```python
from build123d import *

# Parameters (mm, degrees)
SKETCH1_W                                          = 41.91
SKETCH1_H                                          = 101.6
BOSS_EXTRUDE1_DEPTH                                = 41.275
CUT_EXTRUDE6_DEPTH                                 = 78.72202857
SKETCH3_R                                          = 14.3002
CUT_EXTRUDE2_DEPTH                                 = 69.726833551
SKETCH17_W                                         = 28.321
SKETCH17_H                                         = 10.16
CUT_EXTRUDE7_DEPTH                                 = 78.72202857
SKETCH4_R                                          = 3.2258
CUT_EXTRUDE3_DEPTH                                 = 112.648097386
FILLET2_R                                          = 3.175
CSK_FOR_10_FLAT_HEAD_MACHINE_SCREW_100_D           = 5.6134
CSK_FOR_10_FLAT_HEAD_MACHINE_SCREW_100_DEPTH       = 38.1
CSK_FOR_10_FLAT_HEAD_MACHINE_SCREW_100_CSINK_D     = 9.779
CSK_FOR_10_FLAT_HEAD_MACHINE_SCREW_100_CSINK_ANGLE = 100
CSK_FOR_10_FLAT_HEAD_MACHINE_SCREW_100_TIP         = 1.686435499
FILLET3_R                                          = 2.54
FILLET4_R                                          = 1.27


with BuildPart() as part:
    # Sketch1 → Boss-Extrude1 (new body)
    with BuildSketch(Plane(origin=(0, 0, 0), x_dir=(1, 0, 0), z_dir=(0, 1, 0))):
        Rectangle(SKETCH1_W, SKETCH1_H)
    extrude(amount=BOSS_EXTRUDE1_DEPTH)

    # Sketch13 → Cut-Extrude6 (cut, through all)
    with BuildSketch(Plane.ZY.offset(20.955)):
        Polygon((-6.872463407, 34.925), (-12.7, 26.60241523), (-12.7, 13.632261674), (-7.600905481, 6.35), (50.8, 6.35), (50.8, 34.925), align=None)
    extrude(amount=-CUT_EXTRUDE6_DEPTH, mode=Mode.SUBTRACT)

    # Sketch3 → Cut-Extrude2 (cut, through all)
    # profile 1 of 2: a face of its own
    with BuildSketch(Plane(origin=(0, 41.275, 0), x_dir=(1, 0, 0), z_dir=(0, 1, 0))):
        with Locations(Location((0, -25.4, 0), (0, 0, 270))):
            Circle(SKETCH3_R)
        Polygon((5.499261314, -25.4), (2.749630657, -20.6375), (-2.749630657, -20.6375), (-5.499261314, -25.4), (-2.749630657, -30.1625), (2.749630657, -30.1625), align=None, mode=Mode.SUBTRACT)
    # profile 2 of 2: a face of its own
    with BuildSketch(Plane(origin=(0, 41.275, 0), x_dir=(1, 0, 0), z_dir=(0, 1, 0))):
        Polygon((2.749630657, -30.1625), (5.499261314, -25.4), (2.749630657, -20.6375), (-2.749630657, -20.6375), (-5.499261314, -25.4), (-2.749630657, -30.1625), align=None)
    extrude(amount=-CUT_EXTRUDE2_DEPTH, mode=Mode.SUBTRACT)

    # Sketch17 → Cut-Extrude7 (cut, through all)
    with BuildSketch(Plane.ZY.offset(20.955)):
        with Locations((-36.6395, 5.08)):
            Rectangle(SKETCH17_W, SKETCH17_H)
    extrude(amount=-CUT_EXTRUDE7_DEPTH, mode=Mode.SUBTRACT)

    # Sketch4 → Cut-Extrude3 (cut, through all)
    with BuildSketch(Plane(origin=(0, 0, -50.8), x_dir=(-1, 0, 0), z_dir=(0, 0, -1))):
        with Locations((11.1125, 20.6375)):
            Circle(SKETCH4_R)
        with Locations((-11.1125, 20.6375)):
            Circle(SKETCH4_R)
    extrude(amount=-CUT_EXTRUDE3_DEPTH, mode=Mode.SUBTRACT)

    # Fillet2
    fillet2_edges = [part.edges().sort_by_distance(p)[0] for p in [
        (20.955, 3.175, 50.8),
        (-20.955, 3.175, 50.8),
        (0, 10.16, -50.8),
        (0, 10.16, -22.479),
        (0, 0, -22.479),
        (20.955, 38.1, 50.8),
        (-20.955, 38.1, 50.8),
    ]]
    fillet(fillet2_edges, radius=FILLET2_R)

    # CSK for #10 Flat Head Machine Screw (100)4
    with Locations(Plane.XY.offset(-12.7)):
        with Locations((-11.1125, 20.6375), (11.1125, 20.6375)):
            CounterSinkHole(CSK_FOR_10_FLAT_HEAD_MACHINE_SCREW_100_D / 2, CSK_FOR_10_FLAT_HEAD_MACHINE_SCREW_100_CSINK_D / 2, depth=CSK_FOR_10_FLAT_HEAD_MACHINE_SCREW_100_DEPTH, counter_sink_angle=CSK_FOR_10_FLAT_HEAD_MACHINE_SCREW_100_CSINK_ANGLE)
            with Locations((0, 0, -(CSK_FOR_10_FLAT_HEAD_MACHINE_SCREW_100_DEPTH + CSK_FOR_10_FLAT_HEAD_MACHINE_SCREW_100_TIP / 2))):  # 118° drill point
                Cone(0, CSK_FOR_10_FLAT_HEAD_MACHINE_SCREW_100_D / 2, CSK_FOR_10_FLAT_HEAD_MACHINE_SCREW_100_TIP, mode=Mode.SUBTRACT)

    # Fillet3
    fillet3_edges = [part.edges().sort_by_distance(p)[0] for p in [
        (0, 34.925, -6.872463407),
        (0, 6.35, -7.600905481),
    ]]
    fillet(fillet3_edges, radius=FILLET3_R)

    # Fillet4
    fillet4_edges = [part.edges().sort_by_distance(p)[0] for p in [
        (0, 13.632261674, -12.7),
        (0, 26.60241523, -12.7),
    ]]
    fillet(fillet4_edges, radius=FILLET4_R)


solid = part.part
```
Input: part model. Units: mm. Frame: model coordinates. A direction names the side the tool comes from. Give positions to 0.01 mm unless a question says otherwise; leave off trailing zeros. Loops run counter-clockwise (first coordinate to the right, second up) from the corner with the lowest first, then second, coordinate; pieces in that order, holes last.
1) Line query: L1, parallel to X at y = 3, z = 25 (3 decimals); L2, parallel to Y at x = 17, z = 23.5 (3 decimals); L3, parallel to Y at x = -11, z = -38 (3 decimals). Output: solid intervals per line, ascending.
A:
L1: x = -20.955 to -14.295, 14.295 to 20.955
L2: y = 0 to 6.35, 34.925 to 41.275
L3: y = 10.16 to 17.414, 23.861 to 41.275
2) Section query B-B on x = 0. Return the cut outline in (y, z) (3 decimals).
A:
outline: (0, -19.304) arc R3.175 ccw to (3.175, -22.479) - (6.985, -22.479) arc R3.175 cw to (10.16, -25.654) - (10.16, -47.625) arc R3.175 ccw to (13.335, -50.8) - (41.275, -50.8) - (41.275, 11.1) - (34.925, 11.1) - (34.925, -5.55) arc R2.54 cw to (33.842, -7.631) - (26.93, -12.47) arc R1.27 cw to (26.202, -12.7) - (14.033, -12.7) arc R1.27 cw to (13.304, -12.47) - (7.433, -8.359) arc R2.54 cw to (6.35, -6.279) - (6.35, 11.1) - (0, 11.1) - close; (0, 39.7) - (6.35, 39.7) - (6.35, 50.8) - (0, 50.8) - close; (34.925, 39.7) - (41.275, 39.7) - (41.275, 50.8) - (34.925, 50.8) - close
3) Section query A-A on z = 5.5. Return the cut outline in (x, y) (3 decimals), and give its area (3 significant figures).
A:
outline: (-20.955, 0) - (20.955, 0) - (20.955, 6.35) - (-20.955, 6.35) - close; (-20.955, 34.925) - (20.955, 34.925) - (20.955, 41.275) - (-20.955, 41.275) - close
area: 532 mm2
4) Reachability of faces 4 (the cylindrical face through (0.293, 9.205, -23.384)), 5 (the cylindrical face through (0.293, 6.645, -7.467)) from +Z, -Z, +X, -X, +Y, -Y: full face, straight path, thin tool, end or side. Return the list, or none.
A:
face 4: -Z, +X, -X, -Y
face 5: +Z, +X, -X
5) Section query D-D on z = 25.4. Return the cut outline in (x, y) (3 decimals).
A:
outline: (-20.955, 0) - (-14.3, 0) - (-14.3, 6.35) - (-20.955, 6.35) - close; (-20.955, 34.925) - (-14.3, 34.925) - (-14.3, 41.275) - (-20.955, 41.275) - close; (14.3, 0) - (20.955, 0) - (20.955, 6.35) - (14.3, 6.35) - close; (14.3, 34.925) - (20.955, 34.925) - (20.955, 41.275) - (14.3, 41.275) - close
6) Contact query for flat-ended pins moving along their axis: pin 1 (1.5 mm diameter, centred on x = 0, y = 21, fed in from +Z); pin 2 (17.5 mm diameter, centred on x = 0, z = -41, fed in from -Y); pin 3 (4 mm diameter, centred on x = 6.5, y = 5, fed in from -Z). Output: stop coordinate, or through.
A:
pin 1: stops at z = -12.7
pin 2: stops at y = 10.16
pin 3: stops at z = -22.48
7) Section query C-C on y = 36.5. Return the cut outline in (x, z) (3 decimals).
A:
outline: (-20.955, -50.8) - (20.955, -50.8) - (20.955, 47.625) arc R3.175 ccw to (17.78, 50.8) - (-17.78, 50.8) arc R3.175 ccw to (-20.955, 47.625) - close; hole circle Ø28.6 at (0, 25.4)
8) Mould query, pull axis X, two halves, no side actions, for faces 1 (the flat face through (0, 10.16, -37)), 2 (the flat face through (20.955, 30, -12)), 3 (the cylindrical face through (-10.41, 17.49, -32.7)). Classes: released by +X, released by -X, zero draft, split by the parting line, or undercut.
A:
face 1: zero draft
face 2: released by +X
face 3: undercut
